```python
from build123d import *

# Parameters (mm, degrees)
EXTRUDE_1_DEPTH     = 220
SKETCH_2_R          = 4.25
CUT_EXTRUDE_1_DEPTH = 2
SKETCH_3_R          = 2.25
CUT_EXTRUDE_2_DEPTH = 2
SKETCH_4_R          = 2.25
CUT_EXTRUDE_3_DEPTH = 2
SKETCH_5_R          = 2.25
CUT_EXTRUDE_4_DEPTH = 2


with BuildPart() as part:
    # Эскиз1 → Бобышка-Вытянуть1 (new body)
    with BuildSketch(Plane(origin=(0, 0, 0), x_dir=(1, 0, 0), z_dir=(0, 1, 0))):
        Polygon((0, 0), (0, 20), (1, 20), (1, 1), (20, 1), (20, 0), align=None)
    extrude(amount=EXTRUDE_1_DEPTH)

    # Эскиз2 → Вырез-Вытянуть1 (cut, through all)
    with BuildSketch(Plane(origin=(1, 0, 0), x_dir=(0, 0, -1), z_dir=(1, 0, 0))):
        with Locations((10.5, 180)):
            Circle(SKETCH_2_R)
        with Locations((10.5, 120)):
            Circle(SKETCH_2_R)
        with Locations((10.5, 60)):
            Circle(SKETCH_2_R)
    extrude(amount=-CUT_EXTRUDE_1_DEPTH, mode=Mode.SUBTRACT)

    # Эскиз3 → Вырез-Вытянуть2 (cut, through all)
    with BuildSketch(Plane(origin=(1, 0, 0), x_dir=(0, 0, -1), z_dir=(1, 0, 0))):
        with Locations((10.5, 10)):
            Circle(SKETCH_3_R)
    extrude(amount=-CUT_EXTRUDE_2_DEPTH, mode=Mode.SUBTRACT)

    # Эскиз4 → Вырез-Вытянуть3 (cut, through all)
    with BuildSketch(Plane(origin=(1, 0, 0), x_dir=(0, 0, -1), z_dir=(1, 0, 0))):
        with Locations((10.5, 210)):
            Circle(SKETCH_4_R)
    extrude(amount=-CUT_EXTRUDE_3_DEPTH, mode=Mode.SUBTRACT)

    # Эскиз5 → Вырез-Вытянуть4 (cut, through all)
    with BuildSketch(Plane(origin=(0, 0, -1), x_dir=(-1, 0, 0), z_dir=(0, 0, -1))):
        with Locations((-10, 10)):
            Circle(SKETCH_5_R)
        with Locations((-10, 210)):
            Circle(SKETCH_5_R)
    extrude(amount=-CUT_EXTRUDE_4_DEPTH, mode=Mode.SUBTRACT)


solid = part.part
```
Source: CAD feature listing. Evaluate the final solid. Frame: model axes, mm. A direction names the side the tool comes from. Give positions to 0.01 mm unless a question says otherwise; leave off trailing zeros. Write each loop counter-clockwise with the first axis right and the second up, starting at its lowest first coordinate (ties: lowest second). Pieces come first, ordered by that corner, then holes. Notation, with made-up numbers: (-34, 17) - (-28, 17) arc R13 cw to (-28, 39) - close; hole circle Ø8 at (73, 34). An arc over 180 degrees is marked (long way). One line per item, written item: value. Start each with the question number.
Q1. First-contact query: pin 1 Ø1.5 at (x, z) = (2.5, -10) entering from +Y; pin 2 Ø6 at (y, z) = (136, -9.5) entering from +X; pin 3 Ø4 at (x, y) = (10.5, 137) entering from -Z. Flat tips, straight axial feed; report the tip coordinate or a pass-through.
Q2. Set-up query: faces 1 (the face through (5.6, 0, -0.4)), 2 (the face through (10, 108, -1)). Return all of +Z, -Z, +X, -X, +Y, -Y with unobstructed straight access to the full face (end or side cutting, diameter ignored); none if empty.
Q3. Section query A-A, the plane y = 120. Return the cut outline in (x, z), then the cut area to 3 significant figures.
Q4. Draft query along Z for faces 3 (the face through (5.6, 220, -0.4)), 4 (the face through (0.507, 184.214, -9.947)), 5 (the face through (10, 108, 0)), 6 (the face through (0.507, 123.584, -12.785)). Return one class per face: +Z half, -Z half, draft (parallel to the pull), parting line (faces both ways), or undercut.
Q5. Section query B-B, the plane y = 10. Return the cut outline in (x, z).
Q6. Section query D-D, the plane y = 82. Return the cut outline in (x, z).
Q7. Material intervals for probe 1 along Y at (x, z) = (0.4, -10.5); probe 2 along X at (y, z) = (210, -0.55); probe 3 along Z at (x, y) = (8, 53.5), sorted ascending. Write a range as from..to.
Q8. Section query C-C, the plane x = 10. Return the cut outline in (y, z).
Answer:
1. pin 1: passes through
1. pin 2: stops at x = 1
1. pin 3: stops at z = -1
2. face 1: +Z, -Z, +X, -X, -Y
2. face 2: -Z, +X, +Y, -Y
3. outline: (0, -20) - (1, -20) - (1, -14.75) - (0, -14.75) - close; (0, -6.25) - (1, -6.25) - (1, -1) - (20, -1) - (20, 0) - (0, 0) - close
3. area: 30.5 mm2
4. face 3: draft
4. face 4: undercut
4. face 5: +Z half
4. face 6: undercut
5. outline: (0, -20) - (1, -20) - (1, -12.75) - (0, -12.75) - close; (0, -8.25) - (1, -8.25) - (1, -1) - (7.75, -1) - (7.75, 0) - (0, 0) - close; (12.25, -1) - (20, -1) - (20, 0) - (12.25, 0) - close
6. outline: (0, -20) - (1, -20) - (1, -1) - (20, -1) - (20, 0) - (0, 0) - close
7. probe 1: y = 0..7.75, 12.25..55.75, 64.25..115.75, 124.25..175.75, 184.25..207.75, 212.25..220
7. probe 2: x = 0..7.75, 12.25..20
7. probe 3: z = -1..0
8. outline: (0, -1) - (7.75, -1) - (7.75, 0) - (0, 0) - close; (12.25, -1) - (207.75, -1) - (207.75, 0) - (12.25, 0) - close; (212.25, -1) - (220, -1) - (220, 0) - (212.25, 0) - close
